Can you work these out from the model? Positions are in its coordinate system, mm. Coordinates: 2 decimals unless noted, no trailing zeros. Order: outer loops, then holes, each group sorted by start corner. A loop starts at its lowest first (then second) coordinate and runs counter-clockwise, first axis right, second up. Notation, with made-up numbers: (-32, -9) -> (-15, -9) arc R17 cw to (-15, 4) -> close; hole circle Ø7 at (-34.75, -30). An arc over 180 degrees is marked (long way). Use a Markdown table: item, result. Add a question column.
1. If I drill on line 1 along Z through (x, y) = (-36.5, 6.5); line 2 along Z through (x, y) = (3.5, 4); line 3 along X through (y, z) = (3.5, 20.5), over which ranges is the centre line in solid material (lowest first)? Write a range as from..to.
2. For pin 1 Ø1 at (x, z) = (-31.5, -4) entering from +Y; pin 2 Ø5 at (x, z) = (-14.5, 13) entering from +Y; pin 3 Ø4 at (x, z) = (9.5, 13) entering from -Y; pin 4 Ø1.8 at (x, z) = (-42.2, -19.44) entering from -Y, each with a flat end and sliding along its axis, tell me the tip position at first contact or that it passes through.
3. We'd pull the mould along Z, two halves only. Please class faces 1 (the flat face through (-3, 10.5, 33)), 2 (the cylindrical face through (33.699, 6.451, 26.414)), 3 (the flat face through (-15, 3, 13)): pulls with the +Z half, pulls with the -Z half, needs draft (parallel to the pull), parting line crosses it, or undercut.
4. Suppose I cut it at B-B, the plane z = 20. List the corners of the cut face in (x, y) for me, then the cut area to 3 significant figures.
5. Suppose I cut it at C-C, the plane y = 1.5. List the corners of the cut face in (x, z) for me.
6. Suppose I cut it at A-A, the plane x = -4. List the corners of the cut face in (y, z) for me, then the cut area to 3 significant figures.
7. Suppose I cut it at D-D, the plane x = 13. List the corners of the cut face in (y, z) for me, then the cut area to 3 significant figures.
```python
from build123d import *

# Parameters (mm, degrees)
SKETCH_2_W               = 90
SKETCH_2_H               = 60
EXTRUDE_1_DEPTH          = 3
SKETCH_4_R               = 3
SKETCH_4_R_2             = 1.25
EXTRUDE_2_DEPTH          = 8
SKETCH_5_W               = 90
SKETCH_5_H               = 60
SKETCH_5_W_2             = 84
SKETCH_5_H_2             = 54
EXTRUDE_3_DEPTH          = 10
SKETCH_7_R               = 1.5
EXTRUDE_4_DEPTH          = 7
SKETCH_8_R               = 1.5
CUT_EXTRUDE_1_DEPTH      = 7
CUT_EXTRUDE_1_DEPTH_BACK = 7
CHAMFER_1_SIZE           = 2.5
FILLET_1_R               = 3
CUT_EXTRUDE_2_DEPTH      = 9
CHAMFER_2_SIZE           = 1


with BuildPart() as part:
    # Эскиз2 → Бобышка-Вытянуть1 (new body)
    with BuildSketch(Plane(origin=(0, 0, 0), x_dir=(1, 0, 0), z_dir=(0, 1, 0))):
        with Locations((-3.203448276, -4.55862069)):
            Rectangle(SKETCH_2_W, SKETCH_2_H)
    extrude(amount=EXTRUDE_1_DEPTH)

    # Эскиз4 → Бобышка-Вытянуть2 (add)
    with BuildSketch(Plane(origin=(0, 3, 0), x_dir=(1, 0, 0), z_dir=(0, 1, 0))):
        with Locations((-36.468484305, 12.94137931)):
            Circle(SKETCH_4_R)
        with Locations((-36.468484305, 12.94137931)):
            Circle(SKETCH_4_R_2, mode=Mode.SUBTRACT)
        with Locations((-15.468484305, 12.94137931)):
            Circle(SKETCH_4_R)
        with Locations((-15.468484305, 12.94137931)):
            Circle(SKETCH_4_R_2, mode=Mode.SUBTRACT)
        with Locations((-15.468484305, -13.05862069)):
            Circle(SKETCH_4_R)
        with Locations((-15.468484305, -13.05862069)):
            Circle(SKETCH_4_R_2, mode=Mode.SUBTRACT)
        with Locations((-36.468484305, -13.05862069)):
            Circle(SKETCH_4_R)
        with Locations((-36.468484305, -13.05862069)):
            Circle(SKETCH_4_R_2, mode=Mode.SUBTRACT)
        with Locations((9.061587753, -13.05862069)):
            Circle(SKETCH_4_R)
        with Locations((9.061587753, -13.05862069)):
            Circle(SKETCH_4_R_2, mode=Mode.SUBTRACT)
        with Locations((30.061587753, -13.05862069)):
            Circle(SKETCH_4_R)
        with Locations((30.061587753, -13.05862069)):
            Circle(SKETCH_4_R_2, mode=Mode.SUBTRACT)
        with Locations((9.061587753, 12.94137931)):
            Circle(SKETCH_4_R)
        with Locations((9.061587753, 12.94137931)):
            Circle(SKETCH_4_R_2, mode=Mode.SUBTRACT)
        with Locations((30.061587753, 12.94137931)):
            Circle(SKETCH_4_R)
        with Locations((30.061587753, 12.94137931)):
            Circle(SKETCH_4_R_2, mode=Mode.SUBTRACT)
    extrude(amount=EXTRUDE_2_DEPTH)

    # Эскиз5 → Бобышка-Вытянуть3 (add)
    with BuildSketch(Plane(origin=(0, 3, 0), x_dir=(1, 0, 0), z_dir=(0, 1, 0))):
        with Locations((-3.203448276, -4.55862069)):
            Rectangle(SKETCH_5_W, SKETCH_5_H)
        with Locations((-3.203448276, -4.55862069)):
            Rectangle(SKETCH_5_W_2, SKETCH_5_H_2, mode=Mode.SUBTRACT)
    extrude(amount=EXTRUDE_3_DEPTH)

    # Эскиз7 → Бобышка-Вытянуть4 (add)
    with BuildSketch(Plane(origin=(0, 3, 0), x_dir=(1, 0, 0), z_dir=(0, 1, 0))):
        with BuildLine():
            Line((-39.203448276, 19.44137931), (-39.203448276, 22.44137931))
            Line((-39.203448276, 22.44137931), (-45.203448276, 22.44137931))
            Line((-45.203448276, 22.44137931), (-45.203448276, 16.44137931))
            Line((-45.203448276, 16.44137931), (-42.203448276, 16.44137931))
            ThreePointArc((-42.203448276, 16.44137931), (-40.082127932, 17.320058967), (-39.203448276, 19.44137931))
        make_face()
        with Locations((-42.203448276, 19.44137931)):
            Circle(SKETCH_7_R, mode=Mode.SUBTRACT)
        with BuildLine():
            Line((38.796551724, 22.44137931), (32.796551724, 22.44137931))
            Line((32.796551724, 22.44137931), (32.796551724, 19.44137931))
            ThreePointArc((32.796551724, 19.44137931), (33.675231381, 17.320058967), (35.796551724, 16.44137931))
            Line((35.796551724, 16.44137931), (38.796551724, 16.44137931))
            Line((38.796551724, 16.44137931), (38.796551724, 22.44137931))
        make_face()
        with Locations((35.796551724, 19.44137931)):
            Circle(SKETCH_7_R, mode=Mode.SUBTRACT)
        with BuildLine():
            Line((32.796551724, -28.55862069), (32.796551724, -31.55862069))
            Line((32.796551724, -31.55862069), (38.796551724, -31.55862069))
            Line((38.796551724, -31.55862069), (38.796551724, -25.55862069))
            Line((38.796551724, -25.55862069), (35.796551724, -25.55862069))
            ThreePointArc((35.796551724, -25.55862069), (33.675231381, -26.437300346), (32.796551724, -28.55862069))
        make_face()
        with Locations((35.796551724, -28.55862069)):
            Circle(SKETCH_7_R, mode=Mode.SUBTRACT)
        with BuildLine():
            Line((-45.203448276, -31.55862069), (-39.203448276, -31.55862069))
            Line((-39.203448276, -31.55862069), (-39.203448276, -28.55862069))
            ThreePointArc((-39.203448276, -28.55862069), (-40.082127932, -26.437300346), (-42.203448276, -25.55862069))
            Line((-42.203448276, -25.55862069), (-45.203448276, -25.55862069))
            Line((-45.203448276, -25.55862069), (-45.203448276, -31.55862069))
        make_face()
        with Locations((-42.203448276, -28.55862069)):
            Circle(SKETCH_7_R, mode=Mode.SUBTRACT)
    extrude(amount=EXTRUDE_4_DEPTH)

    # Эскиз8 → Вырез-Вытянуть1 (cut, two sides)
    with BuildSketch(Plane(origin=(0, 3, 0), x_dir=(1, 0, 0), z_dir=(0, 1, 0))) as cut_extrude_1_sk:
        with Locations((-42.203448276, 19.44137931)):
            Circle(SKETCH_8_R)
        with Locations((35.796551724, 19.44137931)):
            Circle(SKETCH_8_R)
        with Locations((35.796551724, -28.55862069)):
            Circle(SKETCH_8_R)
        with Locations((-42.203448276, -28.55862069)):
            Circle(SKETCH_8_R)
    extrude(amount=CUT_EXTRUDE_1_DEPTH, mode=Mode.SUBTRACT)
    extrude(cut_extrude_1_sk.sketch, amount=-CUT_EXTRUDE_1_DEPTH_BACK, mode=Mode.SUBTRACT)

    # Фаска1
    chamfer_1_edges = [part.edges().sort_by_distance(p)[0] for p in [
        (34.296551724, 0, 28.55862069),
        (-43.703448276, 0, -19.44137931),
        (-43.703448276, 0, 28.55862069),
        (34.296551724, 0, -19.44137931),
    ]]
    chamfer(chamfer_1_edges, length=CHAMFER_1_SIZE)

    # Скругление1
    fillet_1_edges = [part.edges().sort_by_distance(p)[0] for p in [
        (-48.203448276, 6.5, -25.44137931),
        (41.796551724, 6.5, -25.44137931),
        (41.796551724, 6.5, 34.55862069),
        (-48.203448276, 6.5, 34.55862069),
    ]]
    fillet(fillet_1_edges, radius=FILLET_1_R)

    # Эскиз9 → Вырез-Вытянуть2 (cut)
    with BuildSketch(Plane.XY.offset(34.55862069)):
        with BuildLine():
            Line((-5.703448276, 15.5), (-0.703448276, 15.5))
            ThreePointArc((-0.703448276, 15.5), (0.357211896, 15.060660172), (0.796551724, 14))
            Line((0.796551724, 14), (0.796551724, 12))
            ThreePointArc((0.796551724, 12), (0.357211896, 10.939339828), (-0.703448276, 10.5))
            Line((-0.703448276, 10.5), (-5.703448276, 10.5))
            ThreePointArc((-5.703448276, 10.5), (-6.764108448, 10.939339828), (-7.203448276, 12))
            Line((-7.203448276, 12), (-7.203448276, 14))
            ThreePointArc((-7.203448276, 14), (-6.764108448, 15.060660172), (-5.703448276, 15.5))
        make_face()
    extrude(amount=-CUT_EXTRUDE_2_DEPTH, mode=Mode.SUBTRACT)

    # Фаска2
    chamfer_2_edges = [part.edges().sort_by_distance(p)[0] for p in [
        (-7.203448276, 12.5, 34.55862069),
        (-6.764108448, 10.939339828, 34.55862069),
        (-3.203448276, 10.5, 34.55862069),
        (0.357211896, 10.939339828, 34.55862069),
        (0.796551724, 12.5, 34.55862069),
    ]]
    chamfer(chamfer_2_edges, length=CHAMFER_2_SIZE)


solid = part.part
```
Worked out:
| question | item | result |
|---|---|---|
| 1 | line 1 | z = -25.44..-22.44, -15.94..-14.19, -11.69..-9.94, 10.06..11.81, 14.31..16.06, 31.56..34.56 |
| 1 | line 2 | z = -25.44..-22.44, 31.56..34.56 |
| 1 | line 3 | x = -48.2..-45.2, 38.8..41.8 |
| 2 | pin 1 | stops at y = 3 |
| 2 | pin 2 | stops at y = 11 |
| 2 | pin 3 | stops at y = 0 |
| 2 | pin 4 | passes through |
| 3 | face 1 | needs draft |
| 3 | face 2 | undercut |
| 3 | face 3 | undercut |
| 4 | outline | (-48.2, 0) -> (41.8, 0) -> (41.8, 13) -> (38.8, 13) -> (38.8, 3) -> (-45.2, 3) -> (-45.2, 13) -> (-48.2, 13) -> close |
| 4 | area | 330 mm² |
| 5 | outline | (-48.2, -22.44) arc R3 ccw to (-45.2, -25.44) -> (38.8, -25.44) arc R3 ccw to (41.8, -22.44) -> (41.8, 31.56) arc R3 ccw to (38.8, 34.56) -> (-45.2, 34.56) arc R3 ccw to (-48.2, 31.56) -> close; hole circle Ø5 at (-42.2, -19.44); hole circle Ø5 at (-42.2, 28.56); hole circle Ø5 at (35.8, -19.44); hole circle Ø5 at (35.8, 28.56) |
| 6 | outline | (0, -25.44) -> (13, -25.44) -> (13, -22.44) -> (3, -22.44) -> (3, 31.56) -> (10.5, 31.56) -> (10.5, 33.56) -> (9.5, 34.56) -> (0, 34.56) -> close |
| 6 | area | 232 mm² |
| 7 | outline | (0, -25.44) -> (13, -25.44) -> (13, -22.44) -> (3, -22.44) -> (3, 31.56) -> (13, 31.56) -> (13, 34.56) -> (0, 34.56) -> close |
| 7 | area | 240 mm² |
